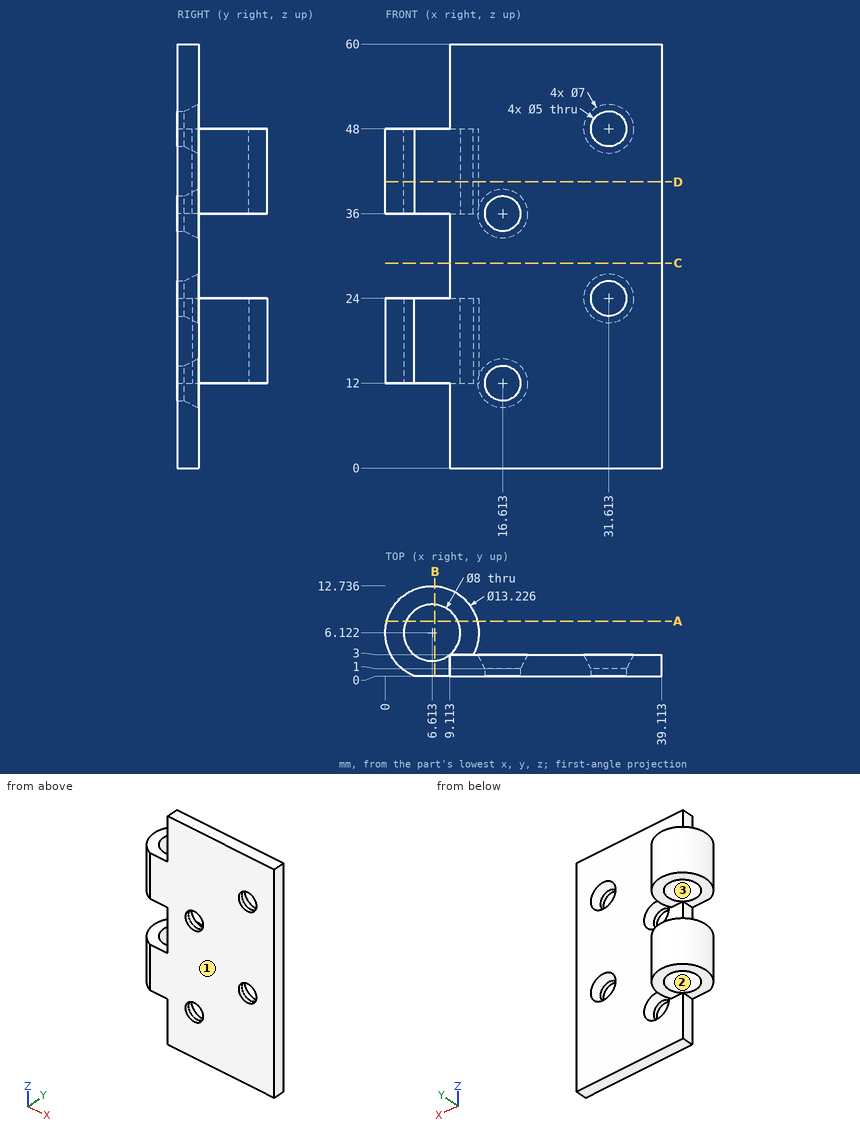
For this review, use the dimensioned drawing (mm, ordinates from the lowest corner) and the shaded views. Give positions to 0.01 mm unless a question says otherwise; leave off trailing zeros. Write each loop counter-clockwise with the first axis right and the second up, starting at its lowest first coordinate (ties: lowest second). Pieces come first, ordered by that corner, then holes.
(1) The part is to be moulded in two halves that separate along Y. For the marked faces 1, 2 and 3, say which applies: released by +Y, released by -Y, zero draft, split by the parting line, or undercut.
(2) Consider section A-A, the plane y = 7.75. Give the boundary of the cut face in (x, z).
(3) Consider section B-B, the plane x = 7. Give the boundary of the cut face in (y, z) (1 decimal).
(4) For P1, Ø1.5, axis at y = 1.5, z = 31.5, coming from the -X side; P2, Ø6, axis at x = 10, z = 14.5, coming from the +Y side (1 decimal); P3, Ø4, axis at x = 6, y = 3.5, coming from the +Z side; P4, Ø4, axis at x = 7.5, y = 5, coming from the +Z side (1 decimal), all flat-tipped, find the tip position at first contact; note any pin that passes through.
(5) Consider section C-C, the plane z = 29. Give the boundary of the cut face in (x, y).
(6) To check wall thickness, follow L1, parallel to Z at x = 9.5, y = 9.25; L2, parallel to Y at x = 23, z = 53; L3, parallel to X at y = 7, z = 45 (1 decimal). State the ranges of each line that lie inside material, in increasing order.
(7) Consider section D-D, the plane z = 40.5. Give the boundary of the cut face in (x, y), and give its area (3 significant figures).
Returned:
1. face 1: released by -Y
1. face 2: undercut
1. face 3: undercut
2. outline: (0.2, 12) - (2.96, 12) - (2.96, 24) - (0.2, 24) - close; (0.2, 36) - (2.96, 36) - (2.96, 48) - (0.2, 48) - close; (10.27, 12) - (13.02, 12) - (13.02, 24) - (10.27, 24) - close; (10.27, 36) - (13.02, 36) - (13.02, 48) - (10.27, 48) - close
3. outline: (0, 12) - (2.1, 12) - (2.1, 24) - (0, 24) - close; (0, 36) - (2.1, 36) - (2.1, 48) - (0, 48) - close; (10.1, 12) - (12.7, 12) - (12.7, 24) - (10.1, 24) - close; (10.1, 36) - (12.7, 36) - (12.7, 48) - (10.1, 48) - close
4. P1: stops at x = 9.11
4. P2: stops at y = 12.7
4. P3: stops at z = 48
4. P4: passes through
5. outline: (9.11, 0) - (39.11, 0) - (39.11, 3) - (9.11, 3) - close
6. L1: z = 12 to 24, 36 to 48
6. L2: y = 0 to 3
6. L3: x = 0.1 to 2.7, 10.5 to 13.2
7. outline: (4.11, 0) - (39.11, 0) - (39.11, 3) - (12.44, 3) arc R6.61 ccw (long way) to start; hole circle Ø8 at (6.61, 6.12)
7. area: 169 mm2
